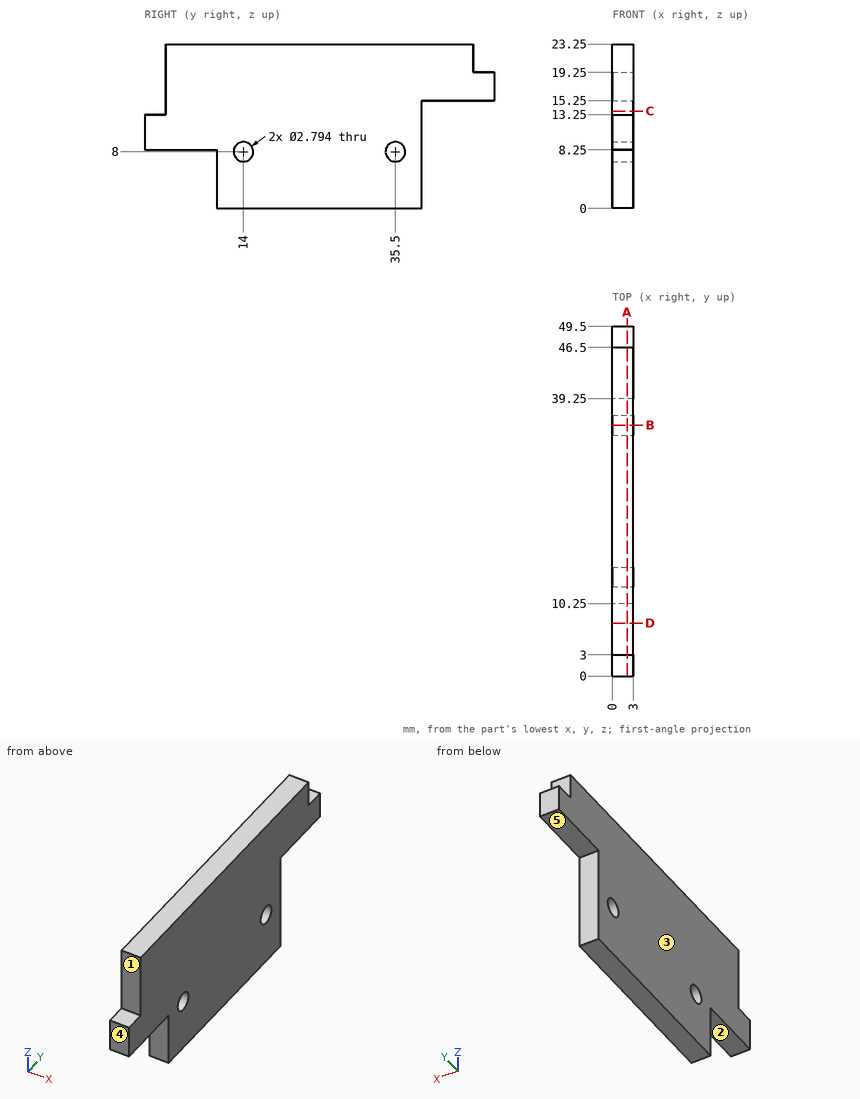
Could you check a few things on this drawing? It's one solid part, dimensions in mm from its lowest x, y, z. A direction names the side the tool comes from. Round coordinates to 2 decimals unless told otherwise and drop trailing zeros. Order: outer loops, then holes, each group sorted by start corner. A loop starts at its lowest first (then second) coordinate and runs counter-clockwise, first axis right, second up.
(1) Which directions (+Z, -Z, +X, -X, +Y, -Y) give clear straight access to the entire face, cutting with the end or side of a thin tool? Please do the marked faces 1, 2, 3, 4 and 5.
Response values:
face 1: +Z, +X, -X, -Y
face 2: -Z, +X, -X, -Y
face 3: +Z, -Z, -X, +Y, -Y
face 4: +Z, -Z, +X, -X, -Y
face 5: -Z, +X, -X, +Y
(2) I'm going to push flat-ended pins straight in: pin 1 (0.9 mm diameter, centred on x = 2, z = 20.5, fed in from +Y); pin 2 (0.9 mm diameter, centred on x = 2, z = 5, fed in from -Y); pin 3 (0.9 mm diameter, centred on x = 1.5, z = 19.5, fed in from -Y); pin 4 (3 mm diameter, centred on y = 14, z = 8, fed in from -X). Where does each tip first touch, or does it pass through?
Response values:
pin 1: stops at y = 46.5
pin 2: stops at y = 10.25
pin 3: stops at y = 3
pin 4: stops at x = 0
(3) Please list where these lines run through material, in increasing order: line 1 along Y through (x, z) = (1.85, 8); line 2 along Y through (x, z) = (0.8, 9); line 3 along Y through (x, z) = (2.35, 14).
Response values:
line 1: y = 10.25 to 12.6, 15.4 to 34.1, 36.9 to 39.25
line 2: y = 0 to 13.02, 14.98 to 34.52, 36.48 to 39.25
line 3: y = 3 to 39.25
(4) Imagine slicing it at C-C (z = 13.75). Write out the boundary of the cut face in (x, y).
Response values:
outline: (0, 3) - (3, 3) - (3, 39.25) - (0, 39.25) - close
(5) Imagine slicing it at D-D (y = 7.5). Write out the boundary of the cut face in (x, z), plus the area to 3 significant figures.
Response values:
outline: (0, 8.25) - (3, 8.25) - (3, 23.25) - (0, 23.25) - close
area: 45.0 mm2
(6) Imagine slicing it at B-B (y = 35.5). Write out the boundary of the cut face in (x, z).
Response values:
outline: (0, 0) - (3, 0) - (3, 6.6) - (0, 6.6) - close; (0, 9.4) - (3, 9.4) - (3, 23.25) - (0, 23.25) - close
(7) Imagine slicing it at A-A (x = 2.1). Write out the boundary of the cut face in (y, z).
Response values:
outline: (0, 8.25) - (10.25, 8.25) - (10.25, 0) - (39.25, 0) - (39.25, 15.25) - (49.5, 15.25) - (49.5, 19.25) - (46.5, 19.25) - (46.5, 23.25) - (3, 23.25) - (3, 13.25) - (0, 13.25) - close; hole circle Ø2.79 at (14, 8); hole circle Ø2.79 at (35.5, 8)
